Read the model definition and answer for the solid it produces. Units are mm, in the model's axes. Give positions to 0.01 mm unless a question says otherwise; leave off trailing zeros. Write each loop counter-clockwise with the first axis right and the second up, starting at its lowest first coordinate (ties: lowest second). Pieces come first, ordered by that corner, then holes. Notation, with made-up numbers: (43, -26.5) -> (72, -26.5) arc R20 ccw to (72, -8.5) -> close; hole circle Ø10 at (-34.75, 65.25). An arc over 180 degrees is marked (long way). Use a Markdown table: item, result.
from build123d import *

# Parameters (mm, degrees)
F0_W     = 114.3
F0_H     = 266.7
F2_DEPTH = 25.4
F1_R     = 12.7
F3_DEPTH = 25.4


with BuildPart() as f2:
    # F0 (on Front) → F2 (new body)
    with BuildSketch(Plane.XZ):
        with Locations((-57.15, 133.35)):
            Rectangle(F0_W, F0_H)
    extrude(amount=F2_DEPTH)

    # F1 (on Front) → F3 (cut)
    with BuildSketch(Plane.XZ):
        with BuildLine():
            ThreePointArc((-44.45, 19.05), (-66.130256, 28.030256), (-57.15, 6.35))
            ThreePointArc((-57.15, 6.35), (-48.169744, 10.069744), (-44.45, 19.05))
        make_face()
        with BuildLine():
            ThreePointArc((-6.35, 19.05), (-28.030256, 28.030256), (-19.05, 6.35))
            ThreePointArc((-19.05, 6.35), (-10.069744, 10.069744), (-6.35, 19.05))
        make_face()
        with Locations((-57.15, 57.15)):
            Circle(F1_R)
        with Locations((-95.25, 57.15)):
            Circle(F1_R)
        with Locations((-19.05, 95.25)):
            Circle(F1_R)
        with Locations((-57.15, 95.25)):
            Circle(F1_R)
        with Locations((-95.25, 133.35)):
            Circle(F1_R)
        with Locations((-57.15, 133.35)):
            Circle(F1_R)
        with Locations((-95.25, 209.55)):
            Circle(F1_R)
        with Locations((-57.15, 209.55)):
            Circle(F1_R)
        with Locations((-19.05, 171.45)):
            Circle(F1_R)
        with Locations((-57.15, 171.45)):
            Circle(F1_R)
        with Locations((-19.05, 247.65)):
            Circle(F1_R)
        with Locations((-57.15, 247.65)):
            Circle(F1_R)
    extrude(amount=F3_DEPTH, mode=Mode.SUBTRACT)


solid = f2.part
Item 1: A cutting plane is placed at B-B (x = -95.25). Give the vertices of the cut face in (y, z).
Return value:
| item | result |
|---|---|
| outline | (-25.4, 0) -> (0, 0) -> (0, 44.45) -> (-25.4, 44.45) -> close; (-25.4, 69.85) -> (0, 69.85) -> (0, 120.65) -> (-25.4, 120.65) -> close; (-25.4, 146.05) -> (0, 146.05) -> (0, 196.85) -> (-25.4, 196.85) -> close; (-25.4, 222.25) -> (0, 222.25) -> (0, 266.7) -> (-25.4, 266.7) -> close |
Item 2: A cutting plane is placed at A-A (z = 247.65). Give the vertices of the cut face in (x, y).
Return value:
| item | result |
|---|---|
| outline | (-114.3, -25.4) -> (-69.85, -25.4) -> (-69.85, 0) -> (-114.3, 0) -> close; (-44.45, -25.4) -> (-31.75, -25.4) -> (-31.75, 0) -> (-44.45, 0) -> close; (-6.35, -25.4) -> (0, -25.4) -> (0, 0) -> (-6.35, 0) -> close |
Item 3: This flat-tipped pin is pushed along its axis until it touches: P1, Ø12, axis at y = -14, z = 173, coming from the +X side. Where does it stop, or does it pass through?
Return value:
| item | result |
|---|---|
| P1 | x = 0 |
Item 4: For a pull along Z with two mould halves and no side action, classify faces 1 (the face through (-45.418, -12.522, 52.286)), 2 (the face through (-114.3, -13, 131)), 3 (the face through (-58, -13, 266.7)) as +Z half, -Z half, draft (parallel to the pull), parting line (faces both ways), or undercut.
Return value:
| item | result |
|---|---|
| face 1 | undercut |
| face 2 | draft |
| face 3 | +Z half |
Item 5: Straight lines are drawn through the part: line 1 along Z through (x, y) = (-95.25, -11); line 2 along Z through (x, y) = (-19.05, -9.75); line 3 along X through (y, z) = (-18.5, 236). For each, find the intervals that lie inside material, in ascending order. Write a range as [from, to].
Return value:
| item | result |
|---|---|
| line 1 | [0, 44.45], [69.85, 120.65], [146.05, 196.85], [222.25, 266.7] |
| line 2 | [0, 6.35], [31.75, 82.55], [107.95, 158.75], [184.15, 234.95], [260.35, 266.7] |
| line 3 | [-114.3, -62.21], [-52.09, -24.11], [-13.99, 0] |
Item 6: A cutting plane is placed at C-C (y = -9.75). Count the separate pieces of the cut face and the enclosed holes in it, then the cut area to 3 significant figures.
Return value:
| item | result |
|---|---|
| separate pieces | 1 |
| enclosed holes | 14 |
| area | 23,400 mm^2 |
Item 7: A cutting plane is placed at D-D (x = -9.5). Give the vertices of the cut face in (y, z), then the cut area to 3 significant figures.
Return value:
| item | result |
|---|---|
| outline | (-25.4, 0) -> (0, 0) -> (0, 10.68) -> (-25.4, 10.68) -> close; (-25.4, 27.42) -> (0, 27.42) -> (0, 86.88) -> (-25.4, 86.88) -> close; (-25.4, 103.62) -> (0, 103.62) -> (0, 163.08) -> (-25.4, 163.08) -> close; (-25.4, 179.82) -> (0, 179.82) -> (0, 239.28) -> (-25.4, 239.28) -> close; (-25.4, 256.02) -> (0, 256.02) -> (0, 266.7) -> (-25.4, 266.7) -> close |
| area | 5,070 mm^2 |
